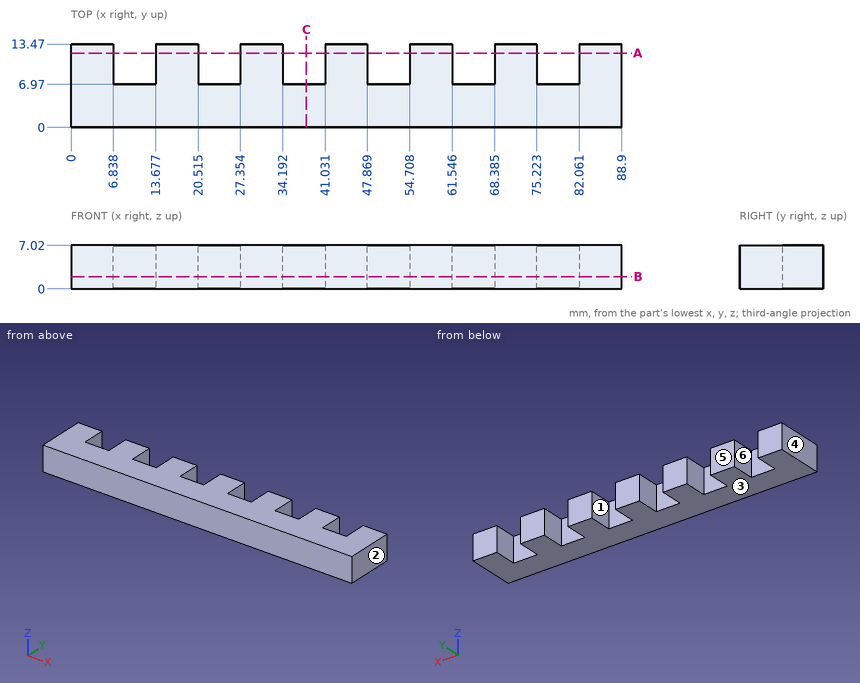
Could you check a few things on this drawing? It's one solid part, dimensions in mm from its lowest x, y, z. A direction names the side the tool comes from. Coordinates: 2 decimals unless noted, no trailing zeros. Write each loop counter-clockwise with the first axis right and the second up, starting at its lowest first coordinate (ties: lowest second). Pieces come first, ordered by that corner, then holes. Notation, with made-up numbers: (23.5, 7) - (54.5, 7) arc R12 cw to (54.5, 22) - close; hole circle Ø10 at (28.5, 63). An arc over 180 degrees is marked (long way). Return JSON: item names as keys, results as strings. Group by question number.
Item 1: Please list where this line runs through material, in increasing order: probe 1 along Y at (x, z) = (39, 4.5).
Item 2: If we section it at C-C (x = 38): Write out the boundary of the cut face in (y, z).
Item 3: Which directions (+Z, -Z, +X, -X, +Y, -Y) give clear straight access to the entire face, cutting with the end or side of a thin tool? Please do the marked faces 5 and 6.
Item 4: If we section it at A-A (y = 12): Write out the boundary of the cut face in (x, z) (1 decimal), then the cut area to 3 significant figures.
Item 5: I'm going to push a flat-ended pin straight in: pin 1 Ø3.5 at (x, z) = (66, 3.5) entering from +Y. Where does the tip first touch, or does it pass through?
Item 6: If we section it at B-B (z = 2): Write out the boundary of the cut face in (x, y) (1 decimal).
Item 7: We'd pull the mould along X, two halves only. Please class the marked faces 1, 2, 3 and 4: pulls with the +X half, pulls with the -X half, needs draft (parallel to the pull), parting line crosses it, or undercut.
Return value:
{
 "1": {"probe 1": "y = 0 to 6.97"},
 "2": {"outline": "(0, 0) - (6.97, 0) - (6.97, 7.02) - (0, 7.02) - close"},
 "3": {"face 5": "+Z, -Z, +X, -X, +Y", "face 6": "+Z, -Z, +Y"},
 "4": {"outline": "(0, 0) - (6.8, 0) - (6.8, 7) - (0, 7) - close; (13.7, 0) - (20.5, 0) - (20.5, 7) - (13.7, 7) - close; (27.4, 0) - (34.2, 0) - (34.2, 7) - (27.4, 7) - close; (41, 0) - (47.9, 0) - (47.9, 7) - (41, 7) - close; (54.7, 0) - (61.5, 0) - (61.5, 7) - (54.7, 7) - close; (68.4, 0) - (75.2, 0) - (75.2, 7) - (68.4, 7) - close; (82.1, 0) - (88.9, 0) - (88.9, 7) - (82.1, 7) - close", "area": "336 mm^2"},
 "5": {"pin 1": "stops at y = 6.97"},
 "6": {"outline": "(0, 0) - (88.9, 0) - (88.9, 13.5) - (82.1, 13.5) - (82.1, 7) - (75.2, 7) - (75.2, 13.5) - (68.4, 13.5) - (68.4, 7) - (61.5, 7) - (61.5, 13.5) - (54.7, 13.5) - (54.7, 7) - (47.9, 7) - (47.9, 13.5) - (41, 13.5) - (41, 7) - (34.2, 7) - (34.2, 13.5) - (27.4, 13.5) - (27.4, 7) - (20.5, 7) - (20.5, 13.5) - (13.7, 13.5) - (13.7, 7) - (6.8, 7) - (6.8, 13.5) - (0, 13.5) - close"},
 "7": {"face 1": "undercut", "face 2": "pulls with the +X half", "face 3": "needs draft", "face 4": "pulls with the -X half"}
}
